Source: CAD feature listing. Evaluate the final solid. Frame: model axes, mm. Give positions to 0.01 mm unless a question says otherwise; leave off trailing zeros. Order: outer loops, then holes, each group sorted by start corner. A loop starts at its lowest first (then second) coordinate and runs counter-clockwise, first axis right, second up.
1) Material intervals for line 1 (X direction, y = 5.25, z = 0.55); line 2 (Y direction, x = 4, z = 0.7); line 3 (X direction, y = 12, z = 0.3), sorted ascending.
2) Section A-A, the plane x = 46. Return loops of the section in (y, z), plus the area to 3 significant figures.
3) Draft query along X for faces 1 (the face through (25, 8, 1)), 2 (the face through (50, 9.9, 0.5)), 3 (the face through (47.42, 4.51, 0.49)). Return one class per face: released by +X, released by -X, zero draft, split by the parting line, or undercut.
4) Section D-D, the plane x = 25. Return loops of the section in (y, z).
5) Section B-B, the plane z = 0.6. Return loops of the section in (x, y).
6) Section C-C, the plane y = 5.25. Return loops of the section in (x, z), plus the area to 3 significant figures.
Autodesk Inventor part; units mm, degrees
ref_plane "YZ Plane" through (0, 0, 0) normal (1, 0, 0) x (0, 1, 0)
ref_plane "XZ Plane" through (0, 0, 0) normal (0, 1, 0) x (-1, 0, 0)
ref_plane "XY Plane" through (0, 0, 0) normal (0, 0, 1) x (1, 0, 0)
sketch "スケッチ1" plane through (0, 0, 0) normal (0, 0, 1) x (1, 0, 0)
  line L0 (0, 0) -> (50, 0)
  line L1 (50, 0) -> (50, 20)
  line L2 (50, 20) -> (0, 20)
  line L3 (0, 20) -> (0, 0)
  dimension "d0" = 20
  dimension "d1" = 50
extrude "押し出し1" add sketch "スケッチ1" along normal blind 1
sketch "スケッチ2" plane through (0, 0, 1) normal (0, 0, 1) x (1, 0, 0)
  line L0 (50, 20) -> (0, 20)
  point P0 (0, 0)
  point P1 (25, 12)
  point P2 (25, 20)
  dimension "d4" = 8
hole "穴1" at (25, 12, 1) direction (0, 0, -1) diameter 4.5 end through all
sketch "スケッチ3" plane through (0, 0, 1) normal (0, 0, 1) x (1, 0, 0)
  line L0 (0, 20) -> (0, 0)
  line L1 (0, 0) -> (50, 0)
  line L2 (50, 20) -> (0, 20)
  point P0 (4, 5.25)
  point P1 (46, 5.25)
  dimension "d12" = 42
  dimension "d13" = 4
  dimension "d22" = 14.75
hole "穴2" at (4, 5.25, 1) at (46, 5.25, 1) direction (0, 0, -1) diameter 3.2 end through all
properties part number "CLS_typeC_31.4N_plate"
From the geometry:
1. line 1: x = 0 to 2.4, 5.6 to 44.4, 47.6 to 50
1. line 2: y = 0 to 3.65, 6.85 to 20
1. line 3: x = 0 to 22.75, 27.25 to 50
2. outline: (0, 0) - (3.65, 0) - (3.65, 1) - (0, 1) - close; (6.85, 0) - (20, 0) - (20, 1) - (6.85, 1) - close
2. area: 16.8 mm2
3. face 1: zero draft
3. face 2: released by +X
3. face 3: undercut
4. outline: (0, 0) - (9.75, 0) - (9.75, 1) - (0, 1) - close; (14.25, 0) - (20, 0) - (20, 1) - (14.25, 1) - close
5. outline: (0, 0) - (50, 0) - (50, 20) - (0, 20) - close; hole circle Ø3.2 at (4, 5.25); hole circle Ø4.5 at (25, 12); hole circle Ø3.2 at (46, 5.25)
6. outline: (0, 0) - (2.4, 0) - (2.4, 1) - (0, 1) - close; (5.6, 0) - (44.4, 0) - (44.4, 1) - (5.6, 1) - close; (47.6, 0) - (50, 0) - (50, 1) - (47.6, 1) - close
6. area: 43.6 mm2
